from build123d import *

# Parameters (mm, degrees)
BOX001_W          = 3.2
BOX001_H          = 8
BOX001_DEPTH      = 10
ARRAY001_COUNT    = 4
CYLINDER001_R     = 50
CYLINDER001_DEPTH = 10
ARRAY_COUNT       = 4
CYLINDER_R        = 23
CYLINDER_DEPTH    = 10
BOX_W             = 120
BOX_H             = 120
BOX_DEPTH         = 3


with BuildPart() as array001:
    # Box001 → Box001 (new body)
    with BuildSketch(Plane(origin=(-1.6, 53, 0), x_dir=(1, 0, 0), z_dir=(0, 0, 1))):
        with Locations((1.6, 4)):
            Rectangle(BOX001_W, BOX001_H)
    extrude(amount=BOX001_DEPTH)

    # Array001: Array001 ×4 about axis
    array001_axis = Axis((0, 0, 0), (0, 0, 1))


with BuildPart() as array001_1:
    add(array001.part)
    for i in range(1, ARRAY001_COUNT):
        add(array001.part.rotate(array001_axis, i * 360 / ARRAY001_COUNT))


with BuildPart() as array:
    # Cylinder001 → Cylinder001 (new body)
    with BuildSketch(Plane(origin=(60, 60, 0), x_dir=(1, 0, 0), z_dir=(0, 0, 1))):
        Circle(CYLINDER001_R)
    extrude(amount=CYLINDER001_DEPTH)

    # Array: Array ×4 about axis
    array_axis = Axis((0, 0, 0), (0, 0, 1))


with BuildPart() as array_1:
    add(array.part)
    for i in range(1, ARRAY_COUNT):
        add(array.part.rotate(array_axis, i * 360 / ARRAY_COUNT))


with BuildPart() as cilindro:
    # Cylinder → Cylinder (new body)
    with BuildSketch(Plane(origin=(60, 60, 0), x_dir=(1, 0, 0), z_dir=(0, 0, 1))):
        Circle(CYLINDER_R)
    extrude(amount=CYLINDER_DEPTH)


with BuildPart() as cut002:
    # Box → Box (new body)
    with BuildSketch(Plane.XY):
        with Locations((60, 60)):
            Rectangle(BOX_W, BOX_H)
    extrude(amount=BOX_DEPTH)

    # Cut: cut Cilindro
    add(cilindro.part, mode=Mode.SUBTRACT)


with BuildPart() as cut002_1:
    # Cut placement: moved
    add(cut002.part.moved(Location((-60, -60, 0))))

    # Cut001: cut Array
    add(array_1.part, mode=Mode.SUBTRACT)

    # Cut002: cut Array001
    add(array001_1.part, mode=Mode.SUBTRACT)


solid = cut002_1.part
Work out the finished part from the listing and answer in its coordinate system (mm). A direction names the side the tool comes from. Give positions to 0.01 mm unless a question says otherwise; leave off trailing zeros. Order: outer loops, then holes, each group sorted by start corner. A loop starts at its lowest first (then second) coordinate and runs counter-clockwise, first axis right, second up. Notation, with made-up numbers: (77.5, 20) - (87.5, 20) arc R18 ccw to (87.5, 33) - close; hole circle Ø4 at (8.5, 17.25). An arc over 180 degrees is marked (long way). Answer as CSV lines item,"result". Start each with the question number.
Q1. The part is cut by section A-A (y = 0). Write down the section's boundary in (x, z).
Q2. The mould has two halves that part along X. Classify faces 1 (the face through (-53, 0, 1)), 2 (the face through (6, 60, 1)), 3 (the face through (-1.6, 56, 1)): +X half, -X half, draft (parallel to the pull), parting line (faces both ways), or undercut.
Q3. The part is cut by section B-B (z = 2.4). Write down the section's boundary in (x, y), then the cut area to 3 significant figures.
Q4. Given pin 1 Ø0.9 at (y, z) = (55.5, 1) entering from -X; pin 2 Ø0.9 at (x, z) = (-0.5, 1) entering from -Y; pin 3 Ø0.9 at (y, z) = (-0.5, 1.5) entering from -X, each flat-ended and moving along its own axis, determine where each tip first touches the part or whether it passes through.
Q5. The part is cut by section D-D (y = 30). Write down the section's boundary in (x, z).
Q6. Find the intervals of material crossed by L1, parallel to X at y = 0, z = 0.7; L2, parallel to Y at x = 54, z = 1.6, in increasing order. Write a range as [from, to].
Q7. For faces 4 (the face through (1.6, 56, 1)), 5 (the face through (56, -1.6, 1)), 6 (the face through (-1.6, -56, 1)), determine the directions among +Z, -Z, +X, -X, +Y, -Y from which every point of the face is accessible in a straight line to the end or side of a thin tool.
Check result:
1,outline,"(-53, 0) - (-23, 0) - (-23, 3) - (-53, 3) - close; (23, 0) - (53, 0) - (53, 3) - (23, 3) - close"
2,face 1,"-X half"
2,face 2,"draft"
2,face 3,"undercut"
3,outline,"(-60, -10) arc R50 cw to (-10, -60) - (-1.6, -60) - (-1.6, -53) - (1.6, -53) - (1.6, -60) - (10, -60) arc R50 cw to (60, -10) - (60, -1.6) - (53, -1.6) - (53, 1.6) - (60, 1.6) - (60, 10) arc R50 cw to (10, 60) - (1.6, 60) - (1.6, 53) - (-1.6, 53) - (-1.6, 60) - (-10, 60) arc R50 cw to (-60, 10) - (-60, 1.6) - (-53, 1.6) - (-53, -1.6) - (-60, -1.6) - close; hole circle Ø46 at (0, 0)"
3,area,"4,790 mm²"
4,pin 1,"stops at x = -10.25"
4,pin 2,"stops at y = -53"
4,pin 3,"stops at x = -53"
5,outline,"(-20, 0) - (20, 0) - (20, 3) - (-20, 3) - close"
6,L1,"x = [-53, -23], [23, 53]"
6,L2,"y = [-10.36, -1.6], [1.6, 10.36]"
7,face 4,"+Z, -Z, +Y"
7,face 5,"+Z, -Z, +X"
7,face 6,"+Z, -Z, -Y"
